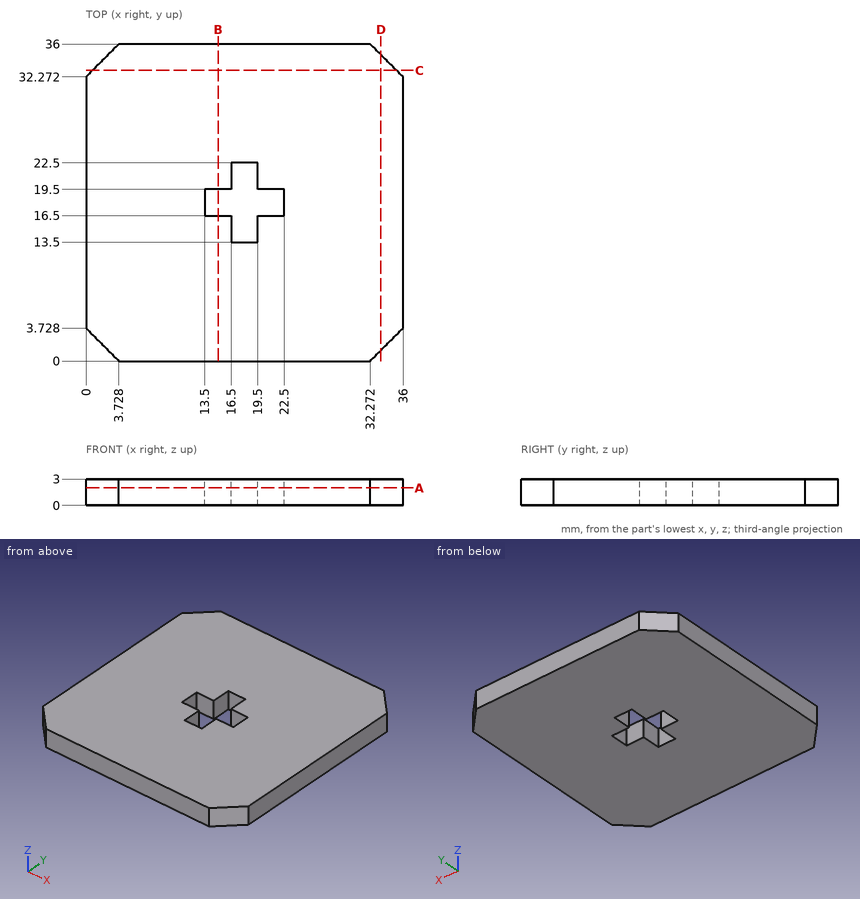
Study the drawing (mm; zero at the part's minimum x, y, z) and answer. Round coordinates to 2 decimals unless told otherwise and drop trailing zeros. Loops run counter-clockwise (first coordinate to the right, second up) from the corner with the lowest first, then second, coordinate; pieces in that order, holes last. Notation, with made-up numbers: M 88,59 L 127,59 A11 ccw 127,80 Z; hole C -24.5,57.5 d5. An arc over 180 degrees is marked long. One line per question, with ' | ' between items.
Q1. Find section A-A, the plane z = 2. Give the vertices of the cut face in (x, y).
Conclusion:
outline: M 0,3.73 L 3.73,0 L 32.27,0 L 36,3.73 L 36,32.27 L 32.27,36 L 3.73,36 L 0,32.27 Z; hole M 13.5,16.5 L 16.5,16.5 L 16.5,13.5 L 19.5,13.5 L 19.5,16.5 L 22.5,16.5 L 22.5,19.5 L 19.5,19.5 L 19.5,22.5 L 16.5,22.5 L 16.5,19.5 L 13.5,19.5 Z
Q2. Find section C-C, the plane y = 33. Give the vertices of the cut face in (x, z).
Conclusion:
outline: M 0.73,0 L 35.27,0 L 35.27,3 L 0.73,3 Z
Q3. This flat-tipped pin is pushed along its axis until it touches: pin 1 Ø0.9 at (x, z) = (21.5, 1.5) entering from -Y. Where does it stop, or does it pass through?
Conclusion:
pin 1: stops at y = 0
Q4. Find section B-B, the plane x = 15. Give the vertices of the cut face in (y, z), then the cut area to 3 significant figures.
Conclusion:
outline: M 0,0 L 16.5,0 L 16.5,3 L 0,3 Z; M 19.5,0 L 36,0 L 36,3 L 19.5,3 Z | area: 99.0 mm2
Q5. Find section D-D, the plane x = 33.5. Give the vertices of the cut face in (y, z), then the cut area to 3 significant figures.
Conclusion:
outline: M 1.23,0 L 34.77,0 L 34.77,3 L 1.23,3 Z | area: 101 mm2
Q6. Consider line 1 along Y through (x, z) = (14.5, 1.1); line 2 along X through (y, z) = (17.5, 2.75). Determine where each line is inside the solid, lowest interval first. Write a range as from..to.
Conclusion:
line 1: y = 0..16.5, 19.5..36 | line 2: x = 0..13.5, 22.5..36
